from build123d import *

# Parameters (mm, degrees)
BOSS_EXTRUDE1_DEPTH = 7
SKETCH2_W           = 9.999992371
SKETCH2_H           = 3.199996948
BOSS_EXTRUDE2_DEPTH = 2
CUT_EXTRUDE1_DEPTH  = 117.710110959


with BuildPart() as part:
    # Sketch1 → Boss-Extrude1 (new body)
    with BuildSketch(Plane.XY.offset(7)):
        Polygon((84.366027832, 79.5), (84.293357849, 79.608764648), (84.207107544, 79.707107544), (84.108764648, 79.79335022), (84, 79.866027832), (83.88269043, 79.923881531), (83.75881958, 79.965927124), (83.630531311, 79.991447449), (83.5, 80), (75.500007629, 80), (75.369476318, 79.991447449), (75.241188049, 79.965927124), (75.1173172, 79.923881531), (75.000007629, 79.866027832), (74.891242981, 79.79335022), (74.792900085, 79.707107544), (74.70664978, 79.608764648), (74.633979797, 79.5), (74.576126099, 79.3826828), (74.534080505, 79.25881958), (74.508560181, 79.130523682), (74.500007629, 79), (74.500007629, 71), (74.508560181, 70.869476318), (74.534080505, 70.74118042), (74.576126099, 70.6173172), (74.633979797, 70.5), (74.70664978, 70.391235352), (74.792900085, 70.292892456), (74.891242981, 70.20664978), (75.000007629, 70.133972168), (75.1173172, 70.076118469), (75.241188049, 70.034072876), (75.369476318, 70.008552551), (75.500007629, 70), (83.5, 70), (83.630531311, 70.008552551), (83.75881958, 70.034072876), (83.88269043, 70.076118469), (84, 70.133972168), (84.108764648, 70.20664978), (84.207107544, 70.292892456), (84.293357849, 70.391235352), (84.366027832, 70.5), (84.423881531, 70.6173172), (84.465927124, 70.74118042), (84.491447449, 70.869476318), (84.5, 71), (84.5, 79), (84.491447449, 79.130523682), (84.465927124, 79.25881958), (84.423881531, 79.3826828), align=None)
    extrude(amount=-BOSS_EXTRUDE1_DEPTH)

    # Sketch2 → Boss-Extrude2 (add)
    with BuildSketch(Plane.XY.offset(7)):
        with Locations((79.500003815, 75)):
            Rectangle(SKETCH2_W, SKETCH2_H)
    extrude(amount=BOSS_EXTRUDE2_DEPTH)

    # Sketch3 → Cut-Extrude1 (cut, through all)
    with BuildSketch(Plane(origin=(0, 0, 0), x_dir=(-1, 0, 0), z_dir=(0, 0, -1))):
        Polygon((-80.454597473, 75.954597473), (-80.669136047, 75.675003052), (-80.804000854, 75.349403381), (-80.850006104, 75), (-80.804000854, 74.650596619), (-80.669136047, 74.324996948), (-80.454597473, 74.045402527), (-80.175003052, 73.830863953), (-79.849411011, 73.695999146), (-79.500007629, 73.650001526), (-79.150596619, 73.695999146), (-78.825004578, 73.830863953), (-78.545410156, 74.045402527), (-78.330871582, 74.324996948), (-78.196006775, 74.650596619), (-78.150001526, 75), (-78.196006775, 75.349403381), (-78.330871582, 75.675003052), (-78.545410156, 75.954597473), (-78.825004578, 76.169136047), (-79.150596619, 76.304000854), (-79.500007629, 76.349998474), (-79.849411011, 76.304000854), (-80.175003052, 76.169136047), align=None)
    extrude(amount=-CUT_EXTRUDE1_DEPTH, mode=Mode.SUBTRACT)


solid = part.part
Geometry: final body of the model. Coordinates: model frame, mm. A direction names the side the tool comes from. Coordinates: 2 decimals unless noted, no trailing zeros. Loops run counter-clockwise (first coordinate to the right, second up) from the corner with the lowest first, then second, coordinate; pieces in that order, holes last. Notation, with made-up numbers: (11.25, 0) - (27.25, 0) arc R25 ccw to (27.25, 21) - close; hole circle Ø2 at (53, -15.75). An arc over 180 degrees is marked (long way). Put each result on its own line as item: value. Start each with the question number.
Q1. Cut plane A-A, the plane z = 8.5. Return loops of the section in (x, y) (3 decimals), and give its area (3 significant figures).
Q2. Cut plane C-C, the plane y = 74.5. Return loops of the section in (x, z).
Q3. Cut plane B-B, the plane x = 76.25. Return loops of the section in (y, z).
Q4. Set-up query: faces 1 (the flat face through (79, 76.6, 8)), 2 (the flat face through (74.5, 75, 4)), 3 (the flat face through (79, 72, 7)). Return all of +Z, -Z, +X, -X, +Y, -Y with unobstructed straight access to the full face (end or side cutting, diameter ignored); none if empty.
Q5. Pin query (flat end, axial travel): pin 1 Ø1 at (x, y) = (81.5, 72.5) entering from +Z; pin 2 Ø0.6 at (x, z) = (82, 8) entering from -Y; pin 3 Ø1 at (x, z) = (81.5, 8) entering from +Y. Return the tip coordinate at first contact, or that it passes through.
Q6. Cut plane D-D, the plane y = 71.75. Return loops of the section in (x, z), and give its area (3 significant figures).
Q7. Line query: line 1 (Z direction, x = 78.25, y = 79.25); line 2 (Y direction, x = 78.25, z = 8); line 3 (Y direction, x = 80.75, z = 0.75). Output: solid intervals per line, ascending.
Filled sheet:
1. outline: (74.5, 73.4) - (84.5, 73.4) - (84.5, 76.6) - (74.5, 76.6) - close; hole (78.15, 75) - (78.196, 74.651) - (78.331, 74.325) - (78.545, 74.045) - (78.825, 73.831) - (79.151, 73.696) - (79.5, 73.65) - (79.849, 73.696) - (80.175, 73.831) - (80.455, 74.045) - (80.669, 74.325) - (80.804, 74.651) - (80.85, 75) - (80.804, 75.349) - (80.669, 75.675) - (80.455, 75.955) - (80.175, 76.169) - (79.849, 76.304) - (79.5, 76.35) - (79.151, 76.304) - (78.825, 76.169) - (78.545, 75.955) - (78.331, 75.675) - (78.196, 75.349) - close
1. area: 26.3 mm²
2. outline: (74.5, 0) - (78.26, 0) - (78.26, 9) - (74.5, 9) - close; (80.74, 0) - (84.5, 0) - (84.5, 9) - (80.74, 9) - close
3. outline: (70, 0) - (80, 0) - (80, 7) - (76.6, 7) - (76.6, 9) - (73.4, 9) - (73.4, 7) - (70, 7) - close
4. face 1: +Z, +X, -X, +Y
4. face 2: +Z, -Z, -X, +Y, -Y
4. face 3: +Z, +X, -X, -Y
5. pin 1: z = 7
5. pin 2: y = 73.4
5. pin 3: y = 76.6
6. outline: (74.5, 0) - (84.5, 0) - (84.5, 7) - (74.5, 7) - close
6. area: 70.0 mm²
7. line 1: 0 to 7
7. line 2: 73.4 to 74.52, 75.48 to 76.6
7. line 3: 70 to 74.52, 75.48 to 80
